Geometry check sheet. Reference: the model listing, model coordinates, mm. Face numbers are marked on the shaded views. A direction names the side the tool comes from. Round coordinates to 2 decimals unless told otherwise and drop trailing zeros. Order: outer loops, then holes, each group sorted by start corner. A loop starts at its lowest first (then second) coordinate and runs counter-clockwise, first axis right, second up. Notation, with made-up numbers: (-4, 87) - (54, 87) arc R23 cw to (54, 124) - close; hole circle Ø1 at (73, -15.5). An arc over 180 degrees is marked (long way). Use a Markdown table: item, result. Add a question column.
(1) Gauge pin test, flat ends, axial feed: P1, Ø4, axis at y = -2, z = 21, coming from the +X side; P2, Ø1.5, axis at x = 16, y = -5, coming from the -Z side; P3, Ø8, axis at x = 17.5, z = 6.5, coming from the -Y side. Record the tip position at first contact, or that the pin passes through.
(2) Section check C-C on z = 28. Record the boundary of the cut face in (x, y).
(3) Section check A-A on x = 5.08. Record the boundary of the cut face in (y, z).
(4) Thickness scan on line 1 along X through (y, z) = (-6.5, 19.5); line 2 along Z through (x, y) = (34, -5.5); line 3 along X through (y, z) = (-4.5, 46.5). Record the ranges inside material, lowest first. Write a range as [from, to].
(5) Access from +Z, -Z, +X, -X, +Y, -Y to the whole of each face (thin tool, end or side, straight path). Record for the marked faces 1 and 2.
(6) Section check D-D on x = 25. Record the boundary of the cut face in (y, z), then the cut area to 3 significant figures.
```python
from build123d import *

# Parameters (mm, degrees)
F1_DEPTH    = 8.89
F2_R        = 3.683
F3_DEPTH    = 13.208
F4_R        = 2.54
F5_T1_DEPTH = 38.1
F6_T1_DEPTH = 47.4109630585


# Not quite as in the source:
# - a fillet or chamfer that OpenCascade refuses, or shapes differently, is made with other operations: its cross-section is extruded or revolved along the edge and cut away or added


with BuildPart() as f1:
    # F0 (on Front) → F1 (new body)
    with BuildSketch(Plane.XZ):
        Polygon((0, 50.8), (0, 0), (10.16, 0), (10.16, 36.405056715), (10.16, 43.18), (17.1377565712, 43.18), (38.1, 43.18), (38.1, 50.8), align=None)
        Polygon((10.16, 43.18), (10.16, 36.405056715), (17.1377565712, 43.18), align=None)
    extrude(amount=F1_DEPTH)

    # F2 (on Front) → F3 (cut)
    with BuildSketch(Plane.XZ):
        with Locations((6.7352303304, 44.409301132)):
            Circle(F2_R)
    extrude(amount=F3_DEPTH, mode=Mode.SUBTRACT)

    # F4
    f4_edges = [f1.edges().sort_by_distance(p)[0] for p in [
        (0, -4.445, 50.8),
        (38.1, -4.445, 43.18),
    ]]
    fillet(f4_edges, radius=F4_R)

    # F5: fillet of radius 5.842 on 2 edges, made by hand

    # F5_s2 → F5_t1 (cut)
    with BuildSketch(Plane.XZ.offset(-14.605)):
        with BuildLine():
            ThreePointArc((0, 5.842), (1.7110821843, 1.7110821843), (5.842, 0))
            Line((5.842, 0), (0, 0))
            Line((0, 0), (0, 5.842))
        make_face()
        with BuildLine():
            ThreePointArc((4.318, 0), (8.4489178157, 1.7110821843), (10.16, 5.842))
            Line((10.16, 5.842), (10.16, 0))
            Line((10.16, 0), (4.318, 0))
        make_face()
    extrude(amount=F5_T1_DEPTH, mode=Mode.SUBTRACT)

    # F6: fillet of radius 5.08 on 1 edges, made by hand

    # F6_s2 → F6_t1 (cut)
    with BuildSketch(Plane.XZ.offset(-19.2604815292)):
        with BuildLine():
            ThreePointArc((0, 5.8419882424), (5.08, 0.7619984664), (10.16, 5.8419882424))
            ThreePointArc((10.16, 5.8419882424), (8.710066706, 1.9898948547), (5.08, 0.0499088405))
            ThreePointArc((5.08, 0.0499088405), (1.449933294, 1.9898948547), (0, 5.8419882424))
        make_face()
    extrude(amount=F6_T1_DEPTH, mode=Mode.SUBTRACT)


solid = f1.part
```
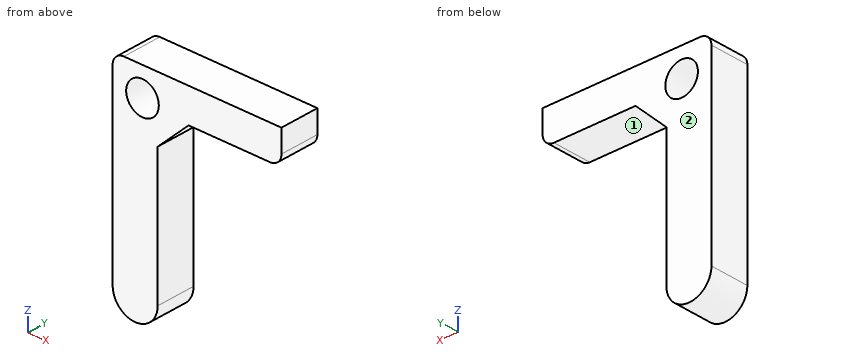
Check sheet entries:
| question | item | result |
|---|---|---|
| 1 | P1 | stops at x = 10.16 |
| 1 | P2 | stops at z = 41.35 |
| 1 | P3 | passes through |
| 2 | outline | (0, -8.89) - (10.16, -8.89) - (10.16, 0) - (0, 0) - close |
| 3 | outline | (-8.89, 0.76) - (0, 0.76) - (0, 41.12) - (-8.89, 41.12) - close; (-8.89, 47.7) - (0, 47.7) - (0, 50.8) - (-8.89, 50.8) - close |
| 4 | line 1 | x = [0, 10.16] |
| 4 | line 2 | z = [43.18, 50.8] |
| 4 | line 3 | x = [0, 3.7], [9.77, 38.1] |
| 5 | face 1 | -Z, +X, +Y, -Y |
| 5 | face 2 | +Z, -Z, +X, -X, +Y |
| 6 | outline | (-8.89, 43.18) - (0, 43.18) - (0, 50.8) - (-8.89, 50.8) - close |
| 6 | area | 67.7 mm2 |
